from build123d import *

# Parameters (mm, degrees)
BOSS_EXTRUDE1_DEPTH     = 575
CHAMFER1_SIZE           = 10.969655115
CHAMFER1_SIZE_2         = 19
FILLET1_R               = 30
CUT_EXTRUDE1_DEPTH      = 250
CUT_EXTRUDE1_DEPTH_BACK = 250
SKETCH3_R               = 16.5
SKETCH4_R               = 7.5
BOSS_EXTRUDE2_DEPTH     = 20
BOSS_EXTRUDE3_START     = 20
SKETCH5_R               = 7.5
BOSS_EXTRUDE3_DEPTH     = 20


with BuildPart() as part:
    # Sketch2 → Boss-Extrude1 (new body)
    with BuildSketch(Plane(origin=(0, 0, 0), x_dir=(0, 0, -1), z_dir=(1, 0, 0))):
        Polygon((-260, 0), (260, 0), (260, 75), (207, 75), (207, 64), (220, 64), (220, 4), (-220, 4), (-220, 64), (-207, 64), (-207, 75), (-260, 75), align=None)
    extrude(amount=-BOSS_EXTRUDE1_DEPTH)

    # Chamfer1
    # the kernel refuses this chamfer: 19, 10.969655115 mm, written as the material it takes off along each edge
    with BuildSketch(Plane(origin=(49.154629338, 75, -207), x_dir=(0, 0.057893862402671324, -0.9983227437537925), z_dir=(-1, 0, 0)), Plane(origin=(49.154629338, 75, 207), x_dir=(0, -0.9983227437537926, -0.057893862402671296), z_dir=(-1, 0, 0))) as chamfer1_piece_1:
        Polygon((CHAMFER1_SIZE * 0.998322743718, CHAMFER1_SIZE * 0.0578938624006), (-CHAMFER1_SIZE_2 * 0.0578938624027, CHAMFER1_SIZE_2 * 0.998322743754), (0, 0), align=None)
    extrude(amount=673.309258677, mode=Mode.SUBTRACT)

    # Fillet1
    fillet1_edges = [part.edges().sort_by_distance(p)[0] for p in [
        (-575, 75, 243),
        (-575, 75, -238.984827557),
    ]]
    fillet(fillet1_edges, radius=FILLET1_R)

    # Sketch3 → Cut-Extrude1 (cut, two sides: drawn at the far end of the back side and taken through both)
    with BuildSketch(Plane.XY.offset(-CUT_EXTRUDE1_DEPTH_BACK)):
        with Locations((-25, 35)):
            Circle(SKETCH3_R)
        with Locations((-69, 35)):
            Circle(SKETCH3_R)
        with Locations((-113, 35)):
            Circle(SKETCH3_R)
        with Locations((-157, 35)):
            Circle(SKETCH3_R)
        with Locations((-201, 35)):
            Circle(SKETCH3_R)
        with Locations((-245, 35)):
            Circle(SKETCH3_R)
        with Locations((-289, 35)):
            Circle(SKETCH3_R)
        with Locations((-333, 35)):
            Circle(SKETCH3_R)
        with Locations((-377, 35)):
            Circle(SKETCH3_R)
        with Locations((-421, 35)):
            Circle(SKETCH3_R)
        with Locations((-465, 35)):
            Circle(SKETCH3_R)
        with Locations((-509, 35)):
            Circle(SKETCH3_R)
        with Locations((-553, 35)):
            Circle(SKETCH3_R)
    extrude(amount=CUT_EXTRUDE1_DEPTH + CUT_EXTRUDE1_DEPTH_BACK, mode=Mode.SUBTRACT)

    # Sketch4 → Boss-Extrude2 (add)
    with BuildSketch(Plane.XY.offset(260)):
        with Locations((-558.68, 50)):
            Circle(SKETCH4_R)
    extrude(amount=BOSS_EXTRUDE2_DEPTH)

    # Sketch5 → Boss-Extrude3 (add)
    with BuildSketch(Plane(origin=(0, 0, -260), x_dir=(-1, 0, 0), z_dir=(0, 0, -1)).offset(BOSS_EXTRUDE3_START)):
        with Locations(Location((558.68, 50, 0), (0, 0, 180))):
            Circle(SKETCH5_R)
    extrude(amount=-BOSS_EXTRUDE3_DEPTH)


solid = part.part
Could you check a few things on this model? Use its own coordinates, in mm. A direction names the side the tool comes from. Give positions to 0.01 mm unless a question says otherwise; leave off trailing zeros. Order: outer loops, then holes, each group sorted by start corner. A loop starts at its lowest first (then second) coordinate and runs counter-clockwise, first axis right, second up. Notation, with made-up numbers: (-30, 37) -> (-25, 37) arc R19 cw to (-25, 51) -> close; hole circle Ø7 at (40, -7). An arc over 180 degrees is marked (long way). Return JSON: item names as keys, results as strings.
1. For pin 1 Ø1 at (x, y) = (-396.5, 27) entering from -Z; pin 2 Ø10 at (x, y) = (-228, 62.5) entering from +Z, each with a flat end and sliding along its axis, tell me the tip position at first contact or that it passes through.
Answer list:
{"pin 1": "stops at z = -260", "pin 2": "stops at z = 260"}
2. On a 3-axis mill with a long thin cutter (end or side, diameter ignored), from which of +Z, -Z, +X, -X, +Y, -Y can I reach the whole of each face in a straight line? I mean faces 1 (the flat face through (-283, 0, 4)), 2 (the flat face through (-157, 35, -250)). Say none if no direction works.
Answer list:
{"face 1": "+Z, -Z, +X, -X, -Y", "face 2": "none"}
3. I need wall thicknesses on line 1 (Z direction, x = -41.5, y = 50.5); line 2 (Z direction, x = -118, y = 32.5); line 3 (Y direction, x = -245, z = 233). Which ranges of each line are inside material? Lowest first, please. Write a range as from..to.
Answer list:
{"line 1": "z = -260..-220, 220..260", "line 2": "z = -260..-250, 250..260", "line 3": "y = 0..18.5, 51.5..75"}
4. Imagine slicing it at B-B on z = -96. List the corners of the cut face in (x, y) for me.
Answer list:
{"outline": "(-575, 0) -> (0, 0) -> (0, 4) -> (-575, 4) -> close"}
5. Thinking about a two-plate mould opening in X: for faces 3 (the cylindrical face through (-72.577, 18.892, -235.21)), 4 (the flat face through (-283, 4, -3)), 5 (the flat face through (-25, 35, 250)), which applies, pulls with the +X half, pulls with the -X half, needs draft (parallel to the pull), parting line crosses it, or undercut?
Answer list:
{"face 3": "undercut", "face 4": "needs draft", "face 5": "undercut"}
